Work out the finished part from the listing and answer in its coordinate system (mm). Face numbers are marked on the shaded views. A direction names the side the tool comes from. Coordinates: 2 decimals unless noted, no trailing zeros. Order: outer loops, then holes, each group sorted by start corner. A loop starts at its lowest first (then second) coordinate and runs counter-clockwise, first axis right, second up. Notation, with made-up numbers: M -12,28 L 16,28 A20 ccw 16,53 Z; hole C 50,-39 d8. An arc over 180 degrees is marked long. Use a Markdown table: item, result.
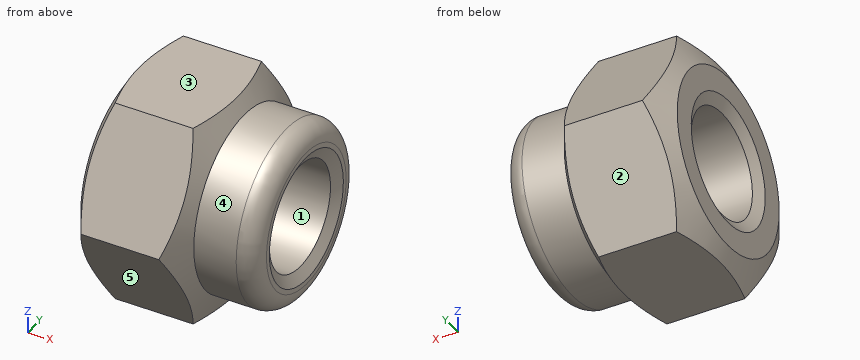
Autodesk Inventor part; units mm, degrees
ref_plane "Work Plane1" through (13.9848, 0, 0) normal (0, 0, 1) x (-1, 0, 0)
ref_plane "YZ Plane" through (0, 0, 0) normal (1, 0, 0) x (0, 1, 0)
ref_plane "XZ Plane" through (0, 0, 0) normal (0, 1, 0) x (-1, 0, 0)
sketch "Sketch1" plane through (0, 0, 0) normal (1, 0, 0) x (0, 1, 0)
  line L0 (2.3094, -4) -> (-2.3094, -4)
  line L1 (-2.3094, -4) -> (-4.6188, 0)
  line L2 (-4.6188, 0) -> (-2.3094, 4)
  line L3 (-2.3094, 4) -> (2.3094, 4)
  line L4 (2.3094, 4) -> (4.6188, 0)
  line L5 (4.6188, 0) -> (2.3094, -4)
  point P0 (0, 0)
  point P1 (0, 0)
  dimension "d0" = 9.2376
extrude "Body" add sketch "Sketch1" along normal blind 4.4
sketch "Sketch2" plane through (4.4, 0, 0) normal (1, 0, 0) x (0, 0, -1)
  circle A0 centre (0, 0) radius 3.44
  dimension "d7" = 6.88
extrude "Ring" add sketch "Sketch2" along normal blind 2.4
sketch "Sketch3" plane through (0, 0, 0) normal (0, 0, 1) x (1, 0, 0)
  line L0 (0, 2.3094) -> (0, 4.6188)
  line L1 (0, 4.6188) -> (4.4, 4.6188)
  line L2 (4.4, 2.3094) -> (4.4, 4.6188)
  line L3 (-0.88, 0) -> (5.28, 0)
  line L4 (0, 3.44) -> (0.6806, 4.6188)
  line L5 (3.7194, 4.6188) -> (4.4, 3.44)
  dimension "d3" = 30
  dimension "d4" = 30
  dimension "d5" = 6.88
  dimension "d6" = 6.88
revolve "Chamfer1" cut sketch "Sketch3" angle 360 about axis through (-10, 0, 0) along (1, 0, 0)
sketch "Sketch4" plane through (0, 0, 0) normal (-1, 0, 0) x (0, 0, 1)
  line L0 (0, -6.4663) -> (0, 6.4663)
  line L1 (-5.6, 0) -> (5.6, 0)
  point P0 (0, 0)
hole "Thread" at (0, 0, 0) direction (1, 0, 0) diameter 4.134 end through all
chamfer "Chamfer2" distance 0.433 angle 30 1 edges at (0, 0, -2.067) measured on face at (0, 2.944, -0.3575)
chamfer "Chamfer3" distance 0.433 angle 30 1 edges at (6.8, 0, -2.067) measured on face at (6.8, -0.2744, -2.949)
ref_plane "Work Plane1" through (13.9848, 0, 0) normal (0, 0, 1) x (-1, 0, 0)
fillet "Fillet1" radius 0.75 1 edges at (6.8, 0, 3.44)
equation "\"d0\" = 1.1547 * SW"
equation "\"d1\" = KOH1"
equation "\"d7\" = SD2"
equation "\"d8\" = KOH - KOH1"
equation "\"d3\" = ANG1"
equation "\"d4\" = ANG2"
equation "\"d5\" = SW0"
equation "\"d6\" = SW01"
equation "\"d10\" = -0.5 * GD1 + 0.5 * NND"
equation "\"d46\" = -0.5 * GD1 + 0.5 * NND"
equation "\"d12\" = -0.5 * GD1 + 0.5 * NND"
equation "\"d47\" = -0.5 * GD1 + 0.5 * NND"
equation "\"ANG1\" = 30deg"
equation "\"ANG2\" = 30deg"
equation "\"NND\" = 5"
equation "\"KOH1\" = 4.4"
equation "\"KOH\" = 6.8"
equation "\"SW\" = 8"
equation "\"SW0\" = 6.88"
equation "\"SW01\" = SW0"
equation "\"SD2\" = SW0"
equation "\"GUL\" = 0.541266 * PTC"
equation "\"THREADDIA\" = 5"
equation "\"TOA\" = 30deg"
equation "\"PTC\" = 0.8"
equation "\"E0\" = 1.155 * SW"
equation "\"GAL\" = 0.541266 * PTC"
properties part number "ISO 7040 - M5" material "Steel"
1. Find the intervals of material crossed by probe 1 along Z at (x, y) = (2.25, 0); probe 2 along Z at (x, y) = (4.75, 0), in increasing order.
Answers below:
| item | result |
|---|---|
| probe 1 | -4 to -2.07, 2.07 to 4 |
| probe 2 | -3.44 to -2.07, 2.07 to 3.44 |
2. For the marked faces 4 and 5, determine the directions among +Z, -Z, +X, -X, +Y, -Y from which every point of the face is accessible in a straight line to the end or side of a thin tool.
Answers below:
| item | result |
|---|---|
| face 4 | +X |
| face 5 | -Z, +X, -X, -Y |
3. Section A-A on x = 3 is taken. Determine the outline of the cut face in (y, z), then the cut area to 3 significant figures.
Answers below:
| item | result |
|---|---|
| outline | M -4.62,0 L -2.31,-4 L 2.31,-4 L 4.62,0 L 2.31,4 L -2.31,4 Z; hole C 0,0 d4.13 |
| area | 42.0 mm² |
4. Section B-B on x = 4.25 is taken. Determine the outline of the cut face in (y, z), then the cut area to 3 significant figures.
Answers below:
| item | result |
|---|---|
| outline | C 0,0 d7.4; hole C 0,0 d4.13 |
| area | 29.6 mm² |
5. A flat-ended cylindrical pin translates along its axis: P1, Ø1, axis at x = 2.5, y = -3, coming from the +Z side. Find the tip coordinate at first contact, or state that the pin passes through.
Answers below:
| item | result |
|---|---|
| P1 | z = 3.67 |
6. For a pull along Y with two mould halves and no side action, classify the marked faces 1, 2 and 3 as +Y half, -Y half, draft (parallel to the pull), parting line (faces both ways), or undercut.
Answers below:
| item | result |
|---|---|
| face 1 | undercut |
| face 2 | +Y half |
| face 3 | draft |
